from build123d import *

# Parameters (mm, degrees)
SKETCH1_W           = 25
SKETCH1_H           = 25
SKETCH1_R           = 1.75
BOSS_EXTRUDE2_DEPTH = 1
SKETCH4_W           = 25
SKETCH4_H           = 26
SKETCH4_R           = 1.75
BOSS_EXTRUDE3_DEPTH = 1


with BuildPart() as part:
    # Sketch1 → Boss-Extrude2 (new body)
    with BuildSketch(Plane.XY):
        Rectangle(SKETCH1_W, SKETCH1_H)
        with Locations((7.5, 2.5)):
            Circle(SKETCH1_R, mode=Mode.SUBTRACT)
        with Locations((-7.5, 7.5)):
            Circle(SKETCH1_R, mode=Mode.SUBTRACT)
    extrude(amount=BOSS_EXTRUDE2_DEPTH)

    # Sketch4 → Boss-Extrude3 (add)
    with BuildSketch(Plane.XZ.offset(12.5)):
        with Locations((0, 13)):
            Rectangle(SKETCH4_W, SKETCH4_H)
        with Locations((7.5, 21)):
            Circle(SKETCH4_R, mode=Mode.SUBTRACT)
        with Locations((-7.5, 16)):
            Circle(SKETCH4_R, mode=Mode.SUBTRACT)
    extrude(amount=BOSS_EXTRUDE3_DEPTH)


solid = part.part
Geometry check sheet. Reference: the model listing, model coordinates, mm. A direction names the side the tool comes from. Give positions to 0.01 mm unless a question says otherwise; leave off trailing zeros. Order: outer loops, then holes, each group sorted by start corner. A loop starts at its lowest first (then second) coordinate and runs counter-clockwise, first axis right, second up. Notation, with made-up numbers: (18, -36) - (23, -36) arc R29 cw to (23, -6) - close; hole circle Ø4 at (61, 54.5). An arc over 180 degrees is marked (long way). Use one line per item in the form item = value.
1) Depth check by flat-ended pin: pin 1 Ø5 at (x, z) = (2, 11.5) entering from +Y; pin 2 Ø12.5 at (x, y) = (-5.5, -5.5) entering from +Z. Enter the tip coordinate at first touch or a pass-through.
Working result:
pin_1 = -12.5
pin_2 = 1
2) Draft check along Y on faces 1 (the face through (0, -13.5, 13)), 2 (the face through (9.117, 1.83, 0.493)), 3 (the face through (12.5, -6.2, 0.4)). Enter one of: released by +Y, released by -Y, zero draft, split by the parting line, or undercut.
Working result:
face_1 = released by -Y
face_2 = undercut
face_3 = zero draft
3) Material ranges on probe 1 along Z at (x, y) = (7.5, -12.9); probe 2 along Y at (x, z) = (10.75, 16.5); probe 3 along Z at (x, y) = (-7.5, -13), recorded low to high. Write a range as from..to.
Working result:
probe_1 = 0..19.25, 22.75..26
probe_2 = -13.5..-12.5
probe_3 = 0..14.25, 17.75..26
4) Sectioned sample at A-A (z = 16). Record the boundary of the cut face in (x, y), and give its area (3 significant figures).
Working result:
outline = (-12.5, -13.5) - (-9.25, -13.5) - (-9.25, -12.5) - (-12.5, -12.5) - close; (-5.75, -13.5) - (12.5, -13.5) - (12.5, -12.5) - (-5.75, -12.5) - close
area = 21.5 mm^2
5) Sectioned sample at D-D (x = -3.5). Record the boundary of the cut face in (y, z).
Working result:
outline = (-13.5, 0) - (12.5, 0) - (12.5, 1) - (-12.5, 1) - (-12.5, 26) - (-13.5, 26) - close
6) Sectioned sample at C-C (y = 7.5). Record the boundary of the cut face in (x, z), and give its area (3 significant figures).
Working result:
outline = (-12.5, 0) - (-9.25, 0) - (-9.25, 1) - (-12.5, 1) - close; (-5.75, 0) - (12.5, 0) - (12.5, 1) - (-5.75, 1) - close
area = 21.5 mm^2
7) Access from +Z, -Z, +X, -X, +Y, -Y to the whole of each face (thin tool, end or side, straight path). Record for faces 4 (the face through (7.272, -12.993, 22.735)), 5 (the face through (0, 0, 1)).
Working result:
face_4 = +Y, -Y
face_5 = +Z, +X, -X, +Y
8) Sectioned sample at B-B (x = -7.5). Record the boundary of the cut face in (y, z).
Working result:
outline = (-13.5, 0) - (5.75, 0) - (5.75, 1) - (-12.5, 1) - (-12.5, 14.25) - (-13.5, 14.25) - close; (-13.5, 17.75) - (-12.5, 17.75) - (-12.5, 26) - (-13.5, 26) - close; (9.25, 0) - (12.5, 0) - (12.5, 1) - (9.25, 1) - close
